Source: CAD feature listing. Evaluate the final solid. Frame: model axes, mm. A direction names the side the tool comes from. Give positions to 0.01 mm unless a question says otherwise; leave off trailing zeros. Write each loop counter-clockwise with the first axis right and the second up, starting at its lowest first coordinate (ties: lowest second). Pieces come first, ordered by that corner, then holes. Notation, with made-up numbers: M 19.5,75 L 45.5,75 A24 ccw 45.5,104 Z; hole C 58,-31 d8. An arc over 180 degrees is marked long. Answer as a JSON object with one key per item and string values. Group by question number.
```python
from build123d import *

# Parameters (mm, degrees)
F0_W     = 90.384428855
F0_H     = 47.2447103821
F0_W_2   = 57.4698699638
F0_H_2   = 18.9575916156
F1_DEPTH = 25.4
F2_DEPTH = 25.4
F3_DEPTH = 12.7


with BuildPart() as f1:
    # F0 (on Front) → F1 (new body, symmetric)
    with BuildSketch(Plane.XZ):
        with Locations((-21.9803575892, 6.2321212608)):
            Rectangle(F0_W, F0_H)
        with Locations((-21.9803575892, 6.2321212608)):
            Rectangle(F0_W_2, F0_H_2, mode=Mode.SUBTRACT)
    extrude(amount=F1_DEPTH, both=True)

    # F2 (add): a face of the model
    f2_faces = [f1.faces().sort_by_distance(p)[0] for p in [
        (-21.9803575892, -25.4, 28.8346035363),
    ]]
    extrude(f2_faces, amount=F2_DEPTH)

    # F3 (add): a face of the model
    f3_faces = [f1.faces().sort_by_distance(p)[0] for p in [
        (-21.9803575892, -50.8, 28.8346035363),
    ]]
    extrude(f3_faces, amount=F3_DEPTH)


solid = f1.part
```
(1) Section B-B, the plane z = 6. Return loops of the section in (x, y), plus the area to 3 significant figures.
(2) Ray query, L1, parallel to X at y = -52.5, z = 5; L2, parallel to Z at x = -45, y = 21.5. Return the intervals inside material, ascending. Write a range as [from, to].
(3) Section C-C, the plane y = -39. Return loops of the section in (x, z).
(4) Section A-A, the plane x = -49. Return loops of the section in (y, z), plus the area to 3 significant figures.
(5) Access query for faces 4 (the flat face through (-23, -18, 29.854)), 5 (the flat face through (6.755, -18, 6)). Directions: +Z, -Z, +X, -X, +Y, -Y. A direction counts if a zero-diameter tool reaches every point of the face in a straight line with its end or side. Return the directions, or none.
(6) Pull-direction query (Z, two-part tool) for faces 1 (the flat face through (-23, -18, -17.39)), 2 (the flat face through (-67.173, -18, 6)), 3 (the flat face through (-22, -18, -3.247)); classes: pulls with the +Z half, pulls with the -Z half, needs draft (parallel to the pull), parting line crosses it, or undercut.
Reported:
{
 "1": {"outline": "M -67.17,-63.5 L -50.72,-63.5 L -50.72,25.4 L -67.17,25.4 Z; M 6.75,-63.5 L 23.21,-63.5 L 23.21,25.4 L 6.75,25.4 Z", "area": "2,930 mm2"},
 "2": {"L1": "x = [-67.17, -50.72], [6.75, 23.21]", "L2": "z = [-17.39, -3.25], [15.71, 29.85]"},
 "3": {"outline": "M -67.17,-17.39 L 23.21,-17.39 L 23.21,29.85 L -67.17,29.85 Z; hole M -50.72,-3.25 L 6.75,-3.25 L 6.75,15.71 L -50.72,15.71 Z"},
 "4": {"outline": "M -63.5,-17.39 L 25.4,-17.39 L 25.4,-3.25 L -63.5,-3.25 Z; M -63.5,15.71 L 25.4,15.71 L 25.4,29.85 L -63.5,29.85 Z", "area": "2,510 mm2"},
 "5": {"face 4": "+Z, +X, -X, +Y, -Y", "face 5": "+Y, -Y"},
 "6": {"face 1": "pulls with the -Z half", "face 2": "needs draft", "face 3": "undercut"}
}
